Build history of the part. All positions in model axes, mm. Face numbers are marked on the shaded views. Give positions to 0.01 mm unless a question says otherwise; leave off trailing zeros. Order: outer loops, then holes, each group sorted by start corner. A loop starts at its lowest first (then second) coordinate and runs counter-clockwise, first axis right, second up. Notation, with made-up numbers: (22, 42) - (54, 42) arc R33 ccw to (54, 76) - close; hole circle Ø7 at (59.25, -23). An arc over 180 degrees is marked (long way). One line per item, written item: value.
Autodesk Inventor part; units mm, degrees
ref_plane "YZ Plane" through (0, 0, 0) normal (1, 0, 0) x (0, 1, 0)
ref_plane "XZ Plane" through (0, 0, 0) normal (0, 1, 0) x (-1, 0, 0)
ref_plane "XY Plane" through (0, 0, 0) normal (0, 0, 1) x (1, 0, 0)
sketch "Sketch5" plane through (0, 0, 0) normal (0, 0, 1) x (1, 0, 0)
  line L0 (-32, -5) -> (32, -5)
  line L1 (32, -5) -> (32, 5)
  line L2 (32, 5) -> (-32, 5)
  line L3 (-32, 5) -> (-32, -5)
  line L4 (-32, -5) -> (32, 5) construction
  line L5 (32, -5) -> (-32, 5) construction
  point P0 (0, 0)
  dimension "d17" = 64
  dimension "d18" = 10
extrude "Extrusion5" add sketch "Sketch5" along normal mid plane 46.5
sketch "Sketch17" plane through (-32, 5, 23.25) normal (0, 1, 0) x (1, 0, 0)
  line L0 (0, 46.5) -> (0, 0)
  line L1 (0, 23.25) -> (10, 23.25)
  line L2 (10, 23.25) -> (10, 10)
  line L3 (10, 10) -> (10, 36.5)
  line L4 (10, 36.5) -> (48, 36.5)
  line L5 (48, 36.5) -> (48, 10)
  line L6 (48, 10) -> (10, 10)
  point P0 (32, 23.25)
  dimension "d84" = 10
  dimension "d85" = 13.25
  dimension "d86" = 26.5
  dimension "d87" = 38
extrude "Extrusion15" cut sketch "Sketch17" against normal blind 5.2
sketch "Sketch18" plane through (-32, -5, 23.25) normal (-1, 0, 0) x (0, 0, 1)
  line L0 (-46.5, 0) -> (-46.5, 10)
  line L1 (0, 10) -> (0, 0)
  line L2 (-46.5, 0) -> (0, 0)
  line L3 (0, 0) -> (0, 1.8)
  line L4 (0, 1.8) -> (-46.5, 1.8)
  line L5 (-46.5, 1.8) -> (-46.5, 0)
  point P0 (-23.25, 5)
  point P1 (0, 1.8)
  point P2 (-46.5, 1.8)
  dimension "d90" = 1.8
extrude "Extrusion16" cut sketch "Sketch18" against normal through all
properties part number "Enclosure-Bottom"
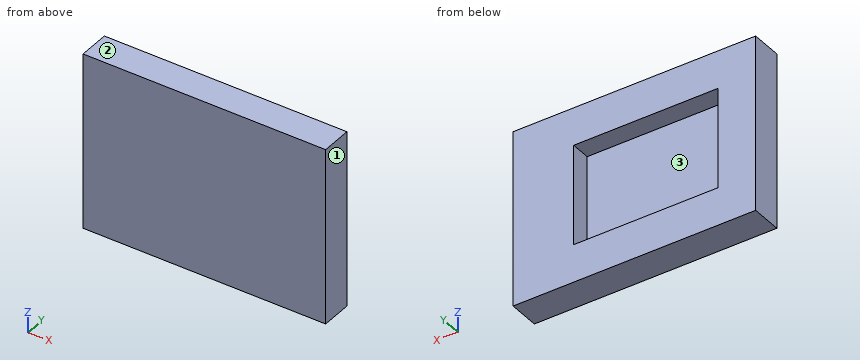
(1) Pull direction X, two halves, no side cores. Call the marked faces 1, 2 and 3: +X half, -X half, draft (parallel to the pull), parting line (faces both ways), or undercut.
Completed:
face 1: +X half
face 2: draft
face 3: undercut
(2) Drill centre lines: line 1 (Z direction, x = -18.5, y = 1); line 2 (X direction, y = 0.5, z = -12.5); line 3 (Y direction, x = -16, z = -5.5). Where is each one in solid material? Low to high.
Completed:
line 1: -23.25 to -13.25, 13.25 to 23.25
line 2: -32 to -22, 16 to 32
line 3: -3.2 to -0.2
(3) Slice it at C-C, the plane x = 13. Give the cut face in (y, z), and give its area (4 significant figures).
Completed:
outline: (-3.2, -23.25) - (5, -23.25) - (5, -13.25) - (-0.2, -13.25) - (-0.2, 13.25) - (5, 13.25) - (5, 23.25) - (-3.2, 23.25) - close
area: 243.5 mm²
(4) Slice it at B-B, the plane z = 10. Give the cut face in (x, y), and give its area (3 significant figures).
Completed:
outline: (-32, -3.2) - (32, -3.2) - (32, 5) - (16, 5) - (16, -0.2) - (-22, -0.2) - (-22, 5) - (-32, 5) - close
area: 327 mm²
(5) Slice it at A-A, the plane y = 3.25. Give the cut face in (x, z).
Completed:
outline: (-32, -23.25) - (32, -23.25) - (32, 23.25) - (-32, 23.25) - close; hole (-22, -13.25) - (16, -13.25) - (16, 13.25) - (-22, 13.25) - close
